Verification items for the finished model (mm, model axes). Face numbers are marked on the shaded views. A direction names the side the tool comes from. Give positions to 0.01 mm unless a question says otherwise; leave off trailing zeros. Write each loop counter-clockwise with the first axis right and the second up, starting at its lowest first coordinate (ties: lowest second). Pieces come first, ordered by that corner, then holes. Notation, with made-up numbers: M 1,-13 L 34,-13 A8 cw 34,-9 Z; hole C 89.5,-35.75 d4. An arc over 180 degrees is marked long. Answer as a JSON object with one key per item and string values.
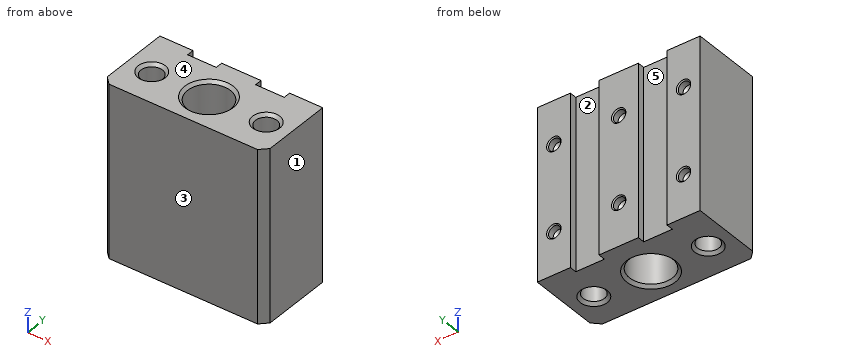
```python
from build123d import *

# Parameters (mm, degrees)
SKETCH_1_W                    = 120.40825663
SKETCH_1_H                    = 69.987299166
EXTRUDE_1_DEPTH               = 30
CUT_EXTRUDE_1_DEPTH           = 98.070897342
CUT_EXTRUDE_1_DEPTH_BACK      = 98.070897342
SKETCH_2_W                    = 9.395515641
SKETCH_2_H                    = 48.745871703
SKETCH_3_W                    = 113.81790299
SKETCH_3_H                    = 30
EXTRUDE_2_DEPTH               = 69.987299167
SKETCH_4_W                    = 113.81790299
SKETCH_4_H                    = 3.825309314
EXTRUDE_3_DEPTH               = 69.987299167
SKETCH_5_W                    = 120
SKETCH_5_H                    = 63.825309314
EXTRUDE_4_DEPTH               = 113.817902989
CUT_EXTRUDE_2_DEPTH           = 148.350937795
CUT_EXTRUDE_2_DEPTH_BACK      = 148.350937795
SKETCH_6_R                    = 15
SKETCH_6_R_2                  = 7.5
CUT_EXTRUDE_3_DEPTH           = 148.350937795
CUT_EXTRUDE_3_DEPTH_BACK      = 148.350937795
SKETCH_7_W                    = 113.81790299
SKETCH_7_H                    = 11.234457722
CUT_EXTRUDE_4_DEPTH           = 148.350937795
CUT_EXTRUDE_4_DEPTH_BACK      = 148.350937795
SKETCH_8_W                    = 20
SKETCH_8_H                    = 5
CHAMFER_1_SIZE                = 5
CHAMFER_2_SIZE                = 2
HOLE_WIZARD_M10_1_D           = 8.5
HOLE_WIZARD_M10_1_DEPTH       = 5
HOLE_WIZARD_M10_1_CSINK_D     = 10.05
HOLE_WIZARD_M10_1_CSINK_ANGLE = 90
HOLE_WIZARD_M10_1_TIP         = 2.553657631


with BuildPart() as part:
    # 草图1 → 凸台-拉伸1 (new body)
    with BuildSketch(Plane(origin=(0, 0, 0), x_dir=(1, 0, 0), z_dir=(0, 1, 0))):
        Rectangle(SKETCH_1_W, SKETCH_1_H)
    extrude(amount=EXTRUDE_1_DEPTH)

    # 草图2 → 切除-拉伸1 (cut, two sides: drawn at the far end of the back side and taken through both)
    with BuildSketch(Plane.XY.offset(34.993649583).offset(-CUT_EXTRUDE_1_DEPTH_BACK)):
        with Locations((-61.606709315, 9.40788871)):
            Rectangle(SKETCH_2_W, SKETCH_2_H)
        Polygon((56.908951495, -11.846624373), (56.908951495, 33.780824562), (63.684524074, 33.780824562), (62.913393862, -11.846624373), align=None)
    extrude(amount=CUT_EXTRUDE_1_DEPTH + CUT_EXTRUDE_1_DEPTH_BACK, mode=Mode.SUBTRACT)

    # 草图3 → 凸台-拉伸2 (add)
    with BuildSketch(Plane.XY.offset(34.993649583)):
        with Locations((0, 45)):
            Rectangle(SKETCH_3_W, SKETCH_3_H)
    extrude(amount=-EXTRUDE_2_DEPTH)

    # 草图4 → 凸台-拉伸3 (add)
    with BuildSketch(Plane.XY.offset(34.993649583)):
        with Locations((0, 61.912654657)):
            Rectangle(SKETCH_4_W, SKETCH_4_H)
    extrude(amount=-EXTRUDE_3_DEPTH)

    # 草图5 → 凸台-拉伸4 (add)
    with BuildSketch(Plane(origin=(56.908951495, 0, 0), x_dir=(0, 0, -1), z_dir=(1, 0, 0))):
        with Locations((25.006350417, 31.912654657)):
            Rectangle(SKETCH_5_W, SKETCH_5_H)
    extrude(amount=-EXTRUDE_4_DEPTH)

    # 草图6 → 切除-拉伸2 (cut, two sides: drawn at the far end of the back side and taken through both)
    with BuildSketch(Plane.XY.offset(34.993649583).offset(-CUT_EXTRUDE_2_DEPTH_BACK)):
        with Locations((0, 33.825309314)):
            Circle(SKETCH_6_R)
        with Locations((-40, 33.825309314)):
            Circle(SKETCH_6_R_2)
        with Locations((40, 33.825309314)):
            Circle(SKETCH_6_R_2)
    extrude(amount=CUT_EXTRUDE_2_DEPTH + CUT_EXTRUDE_2_DEPTH_BACK, mode=Mode.SUBTRACT)

    # 草图7 → 切除-拉伸3 (cut, two sides: drawn at the far end of the back side and taken through both)
    with BuildSketch(Plane.XY.offset(34.993649583).offset(-CUT_EXTRUDE_3_DEPTH_BACK)):
        with Locations((0, 4.382771139)):
            Rectangle(SKETCH_7_W, SKETCH_7_H)
    extrude(amount=CUT_EXTRUDE_3_DEPTH + CUT_EXTRUDE_3_DEPTH_BACK, mode=Mode.SUBTRACT)

    # 草图8 → 切除-拉伸4 (cut, two sides: drawn at the far end of the back side and taken through both)
    with BuildSketch(Plane.XY.offset(34.993649583).offset(-CUT_EXTRUDE_4_DEPTH_BACK)):
        with Locations((-23.75, 61.325309314)):
            Rectangle(SKETCH_8_W, SKETCH_8_H)
        with Locations((23.75, 61.325309314)):
            Rectangle(SKETCH_8_W, SKETCH_8_H)
    extrude(amount=CUT_EXTRUDE_4_DEPTH + CUT_EXTRUDE_4_DEPTH_BACK, mode=Mode.SUBTRACT)

    # 倒角1
    chamfer_1_edges = [part.edges().sort_by_distance(p)[0] for p in [
        (-56.908951495, 10, -25.006350417),
        (56.908951495, 10, -25.006350417),
    ]]
    chamfer(chamfer_1_edges, length=CHAMFER_1_SIZE)

    # 倒角2
    chamfer_2_edges = [part.edges().sort_by_distance(p)[0] for p in [
        (32.5, 33.825309314, -85.006350417),
        (32.5, 33.825309314, 34.993649583),
        (-47.5, 33.825309314, -85.006350417),
        (-47.5, 33.825309314, 34.993649583),
        (-15, 33.825309314, -85.006350417),
        (-15, 33.825309314, 34.993649583),
    ]]
    chamfer(chamfer_2_edges, length=CHAMFER_2_SIZE)

    # M10 螺纹孔1
    with Locations(Plane(origin=(0, 63.825309314, 0), x_dir=(1, 0, 0), z_dir=(0, 1, 0))):
        with Locations((-45.329475747, 55.006350417), (-45.329475747, -4.993649583), (0, -4.993649583), (45.329475747, -4.993649583), (45.329475747, 55.006350417), (0, 55.006350417)):
            CounterSinkHole(HOLE_WIZARD_M10_1_D / 2, HOLE_WIZARD_M10_1_CSINK_D / 2, depth=HOLE_WIZARD_M10_1_DEPTH, counter_sink_angle=HOLE_WIZARD_M10_1_CSINK_ANGLE)
            with Locations((0, 0, -(HOLE_WIZARD_M10_1_DEPTH + HOLE_WIZARD_M10_1_TIP / 2))):  # 118° drill point
                Cone(0, HOLE_WIZARD_M10_1_D / 2, HOLE_WIZARD_M10_1_TIP, mode=Mode.SUBTRACT)


solid = part.part
```
1) Access from +Z, -Z, +X, -X, +Y, -Y to the whole of each face (thin tool, end or side, straight path). Record for the marked faces 4 and 5.
Completed:
{"face 4": "+Z, +X, -X, +Y, -Y", "face 5": "+Z, -Z, +Y"}
2) Section check A-A on z = -75.5. Record the boundary of the cut face in (x, y), and give its area (3 significant figures).
Completed:
{"outline": "M -56.91,15 L -51.91,10 L 51.91,10 L 56.91,15 L 56.91,63.83 L 33.75,63.83 L 33.75,58.83 L 13.75,58.83 L 13.75,63.83 L -13.75,63.83 L -13.75,58.83 L -33.75,58.83 L -33.75,63.83 L -56.91,63.83 Z; hole C -40,33.83 d15; hole C 0,33.83 d30; hole C 40,33.83 d15", "area": "4,840 mm2"}
3) Thickness scan on L1, parallel to Z at x = 0, y = 60.95; L2, parallel to X at y = 61.5, z = 9.5; L3, parallel to X at y = 37, z = -30.5. Record the ranges inside material, lowest first.
Completed:
{"L1": "z = -85.01 to -59.26, -50.76 to 0.74, 9.24 to 34.99", "L2": "x = -56.91 to -33.75, -13.75 to 13.75, 33.75 to 56.91", "L3": "x = -56.91 to -46.79, -33.21 to -14.66, 14.66 to 33.21, 46.79 to 56.91"}
4) Release check for a two-part mould opening along X. For the marked faces 1, 2 and 3 record: pulls with the +X half, pulls with the -X half, needs draft (parallel to the pull), parting line crosses it, or undercut.
Completed:
{"face 1": "pulls with the +X half", "face 2": "undercut", "face 3": "needs draft"}
5) Go/stop test with flat-tipped pins: pin 1 (16 mm diameter, centred on x = -26, z = -23, fed in from +Y); pin 2 (7 mm diameter, centred on x = 45.33, z = 4.99, fed in from +Y). Record where each tip stops, or that it passes through.
Completed:
{"pin 1": "stops at y = 63.83", "pin 2": "stops at y = 58.38"}
